Geometry check sheet. Reference: the model listing, model coordinates, mm. A direction names the side the tool comes from. Coordinates: 2 decimals unless noted, no trailing zeros. Loops run counter-clockwise (first coordinate to the right, second up) from the corner with the lowest first, then second, coordinate; pieces in that order, holes last. Notation, with made-up numbers: (13.25, 54) -> (72.25, 54) arc R32 cw to (72.25, 89) -> close; hole circle Ø7 at (5.5, -38.5). An arc over 180 degrees is marked (long way). Answer as a JSON object with one key per item and string values.
from build123d import *

# Parameters (mm, degrees)
ESQUISSE1_R             = 3.7
ESQUISSE1_R_2           = 3.2
BOSS_EXTRU_1_DEPTH      = 10
ENL_V_START             = -10
ENL_V_MAT_EXTRU_1_DEPTH = 29.708286934
SYM_TRIE2_START         = -10
SYM_TRIE2_COPY_1_DEPTH  = 29.708286934
CONG_1_R                = 2
ESQUISSE3_W             = 16.438795986
ESQUISSE3_H             = 1.5
ESQUISSE3_W_2           = 21.038627968
ENL_V_MAT_EXTRU_2_DEPTH = 19.708286934


with BuildPart() as part:
    # Esquisse1 → Boss.-Extru.1 (new body)
    with BuildSketch(Plane.XY):
        with BuildLine():
            ThreePointArc((5, 10), (0, 15), (-5, 10))
            Line((-5, 10), (-5, -10))
            ThreePointArc((-5, -10), (0, -15), (5, -10))
            Line((5, -10), (5, 10))
        make_face()
        with Locations((0, 10)):
            Circle(ESQUISSE1_R, mode=Mode.SUBTRACT)
        Circle(ESQUISSE1_R_2, mode=Mode.SUBTRACT)
        with Locations((0, -10)):
            Circle(ESQUISSE1_R, mode=Mode.SUBTRACT)
    extrude(amount=BOSS_EXTRU_1_DEPTH)

    # Esquisse2 → Enlèv. mat.-Extru.1 (cut)
    with BuildSketch(Plane.XY.offset(10).offset(ENL_V_START)):
        Polygon((52.761287706, 43.570965779), (5, 7.75), (1, 4.75), (5, 1.75), (52.761287706, -34.070965779), (172.164506969, -34.070965779), (172.164506969, 43.570965779), align=None)
    enl_v_mat_extru_1 = extrude(amount=ENL_V_MAT_EXTRU_1_DEPTH, mode=Mode.SUBTRACT)

    # Symétrie1: Enlèv. mat.-Extru.1 across plane
    add(enl_v_mat_extru_1.mirror(Plane(origin=(0, 0, 0), x_dir=(0, 0, 1), z_dir=(1, 0, 0))), mode=Mode.SUBTRACT)

    # Symétrie2: Enlèv. mat.-Extru.1 across plane
    add(enl_v_mat_extru_1.mirror(Plane.ZX), mode=Mode.SUBTRACT)

    # Symétrie2 copy 1 sketch → Symétrie2 copy 1 (cut)
    with BuildSketch(Plane(origin=(0, 0, 10), x_dir=(-1, 0, 0), z_dir=(0, 0, 1)).offset(SYM_TRIE2_START)):
        Polygon((52.761287706, 43.570965779), (5, 7.75), (1, 4.75), (5, 1.75), (52.761287706, -34.070965779), (172.164506969, -34.070965779), (172.164506969, 43.570965779), align=None)
    extrude(amount=SYM_TRIE2_COPY_1_DEPTH, mode=Mode.SUBTRACT)

    # Congé1
    cong_1_edges = [part.edges().sort_by_distance(p)[0] for p in [
        (1, 4.75, 5),
        (-1, 4.75, 5),
        (-1, -4.75, 5),
        (1, -4.75, 5),
    ]]
    fillet(cong_1_edges, radius=CONG_1_R)

    # Esquisse3 → Enlèv. mat.-Extru.2 (cut, through all)
    with BuildSketch(Plane(origin=(0, 0, 0), x_dir=(-1, 0, 0), z_dir=(0, 0, -1))):
        with Locations((0, 15)):
            Rectangle(ESQUISSE3_W, ESQUISSE3_H)
        with Locations((0, -15)):
            Rectangle(ESQUISSE3_W_2, ESQUISSE3_H)
    extrude(amount=-ENL_V_MAT_EXTRU_2_DEPTH, mode=Mode.SUBTRACT)


solid = part.part
1. Section check B-B, the plane x = -0.5. Record the boundary of the cut face in (y, z).
Evaluation:
{"outline": "(-14.25, 0) -> (-13.67, 0) -> (-13.67, 10) -> (-14.25, 10) -> close; (-6.33, 0) -> (-3.16, 0) -> (-3.16, 10) -> (-6.33, 10) -> close; (3.16, 0) -> (6.33, 0) -> (6.33, 10) -> (3.16, 10) -> close; (13.67, 0) -> (14.25, 0) -> (14.25, 10) -> (13.67, 10) -> close"}
2. Depth check by flat-ended pin: P1, Ø6, axis at y = -4.5, z = 8, coming from the +X side. Enter the tip coordinate at first touch or a pass-through.
Evaluation:
{"P1": "stops at x = 5"}
3. Section check A-A, the plane y = 0. Record the boundary of the cut face in (x, z).
Evaluation:
{"outline": "(-5, 0) -> (-3.2, 0) -> (-3.2, 10) -> (-5, 10) -> close; (3.2, 0) -> (5, 0) -> (5, 10) -> (3.2, 10) -> close"}
4. Section check D-D, the plane y = 11.25. Record the boundary of the cut face in (x, z), then the cut area to 3 significant figures.
Evaluation:
{"outline": "(-4.84, 0) -> (-3.48, 0) -> (-3.48, 10) -> (-4.84, 10) -> close; (3.48, 0) -> (4.84, 0) -> (4.84, 10) -> (3.48, 10) -> close", "area": "27.2 mm^2"}
5. Mould release check, pull along Y, two halves, no side actions. Record for faces 4 (the face through (0, 14.25, 5)), 5 (the face through (-2.539, -1.947, 4.93)), 6 (the face through (5, 9, 5)): released by +Y, released by -Y, zero draft, split by the parting line, or undercut.
Evaluation:
{"face 4": "released by +Y", "face 5": "undercut", "face 6": "zero draft"}
6. Section check C-C, the plane z = 4.5. Record the boundary of the cut face in (x, y).
Evaluation:
{"outline": "(-5, -10) arc R5 ccw to (-2.63, -14.25) -> (2.63, -14.25) arc R5 ccw to (5, -10) -> (5, -7.75) -> (3.13, -6.35) arc R2 cw to (3.13, -3.15) -> (5, -1.75) -> (5, 1.75) -> (3.13, 3.15) arc R2 cw to (3.13, 6.35) -> (5, 7.75) -> (5, 10) arc R5 ccw to (2.63, 14.25) -> (-2.63, 14.25) arc R5 ccw to (-5, 10) -> (-5, 7.75) -> (-3.13, 6.35) arc R2 cw to (-3.13, 3.15) -> (-5, 1.75) -> (-5, -1.75) -> (-3.13, -3.15) arc R2 cw to (-3.13, -6.35) -> (-5, -7.75) -> close; hole circle Ø7.4 at (0, -10); hole circle Ø7.4 at (0, 10); hole circle Ø6.4 at (0, 0)"}
7. Thickness scan on probe 1 along Y at (x, z) = (0, 7); probe 2 along Y at (x, z) = (-4.25, 1); probe 3 along Y at (x, z) = (-1.75, 6.25). Record the ranges inside material, lowest first. Write a range as from..to.
Evaluation:
{"probe 1": "y = -14.25..-13.7, -6.3..-3.2, 3.2..6.3, 13.7..14.25", "probe 2": "y = -12.63..-7.19, -2.31..2.31, 7.19..12.63", "probe 3": "y = -14.25..-13.26, -6.74..-2.68, 2.68..6.74, 13.26..14.25"}
8. Tool access check on faces 1 (the face through (-4, 7, 5)), 2 (the face through (-5, 0, 5)), 3 (the face through (4, 7, 5)). Record the directions out of +Z, -Z, +X, -X, +Y, -Y that give a thin tool (end or side, any length) a straight path to the whole face; none if there is none.
Evaluation:
{"face 1": "+Z, -Z, -X", "face 2": "+Z, -Z, -X, +Y, -Y", "face 3": "+Z, -Z, +X"}
